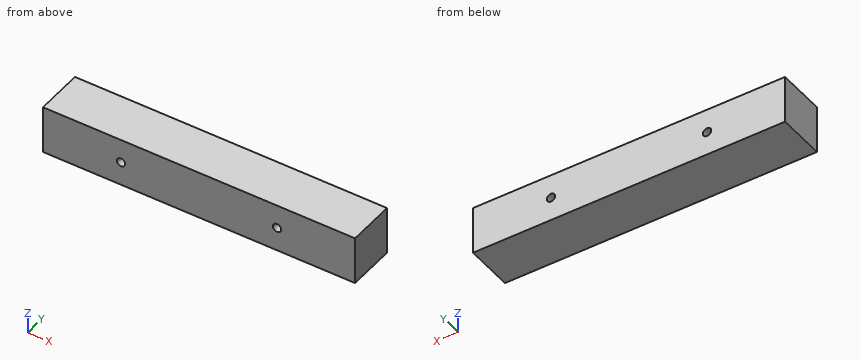
Autodesk Inventor part; units mm, degrees
ref_plane "YZ Plane" through (0, 0, 0) normal (1, 0, 0) x (0, 1, 0)
ref_plane "XZ Plane" through (0, 0, 0) normal (0, 1, 0) x (-1, 0, 0)
ref_plane "XY Plane" through (0, 0, 0) normal (0, 0, 1) x (1, 0, 0)
sketch "스케치2" plane through (0, 0, 0) normal (0, 1, 0) x (-1, 0, 0)
  line L0 (65, 10) -> (-65, 10)
  line L1 (-65, 10) -> (-65, -10)
  line L2 (-65, -10) -> (65, -10)
  line L3 (65, -10) -> (65, 10)
  line L4 (65, 10) -> (-65, -10) construction
  line L5 (-65, 10) -> (65, -10) construction
  point P0 (0, 0)
  dimension "d2" = 130
  dimension "d4" = 20
extrude "돌출2" add sketch "스케치2" along normal blind 20
sketch "스케치3" plane through (0, 20, 0) normal (0, 1, 0) x (1, 0, 0)
  point P0 (0, 0)
  point P1 (32.5, 0)
  point P2 (-32.5, 0)
  dimension "d7" = 32.5
  dimension "d8" = 32.5
hole "구멍1" at (32.5, 20, 0) at (-32.5, 20, 0) direction (0, -1, 0) diameter 3.5 end through all
properties part number "3D지지대"
Input: part model. Units: mm. Frame: model coordinates. Give positions to 0.01 mm unless a question says otherwise; leave off trailing zeros. Order: outer loops, then holes, each group sorted by start corner. A loop starts at its lowest first (then second) coordinate and runs counter-clockwise, first axis right, second up. Notation, with made-up numbers: M 82.5,-18 L 135.5,-18 A32 cw 135.5,20 Z; hole C 41,68.25 d1. An arc over 180 degrees is marked long. One line per question, with ' | ' between items. Start each with the question number.
1. Section query A-A (x = 32.5). Return the cut outline in (y, z), and give its area (3 significant figures).
2. Section query B-B (z = 0). Return the cut outline in (x, y).
3. Material intervals for probe 1 along X at (y, z) = (11.75, 0); probe 2 along Z at (x, y) = (-32.5, 11); probe 3 along X at (y, z) = (9.75, -1.5), sorted ascending. Write a range as [from, to].
Here are the results:
1) outline: M 0,-10 L 20,-10 L 20,-1.75 L 0,-1.75 Z; M 0,1.75 L 20,1.75 L 20,10 L 0,10 Z | area: 330 mm²
2) outline: M -65,0 L -34.25,0 L -34.25,20 L -65,20 Z; M -30.75,0 L 30.75,0 L 30.75,20 L -30.75,20 Z; M 34.25,0 L 65,0 L 65,20 L 34.25,20 Z
3) probe 1: [-65, -34.25], [-30.75, 30.75], [34.25, 65] | probe 2: [-10, -1.75], [1.75, 10] | probe 3: [-65, -33.4], [-31.6, 31.6], [33.4, 65]
